Verification items for the finished model (mm, model axes). A direction names the side the tool comes from. Coordinates: 2 decimals unless noted, no trailing zeros. Order: outer loops, then holes, each group sorted by start corner. A loop starts at its lowest first (then second) coordinate and runs counter-clockwise, first axis right, second up. Notation, with made-up numbers: M 48,51 L 54,51 A10 ccw 54,66 Z; hole C 66,-8 d8. An arc over 180 degrees is marked long. Return JSON: item names as keys, results as strings. Group by question number.
1. Set-up check for faces 1 (the cylindrical face through (-0.867, -3.905, 69.451)), 2 (the cylindrical face through (-6.466, -2.681, 1.972)): record each of +Z, -Z, +X, -X, +Y, -Y from which the full face is reachable in a straight line by a thin tool's end or side.
2. Section check D-D, the plane z = 61. Record the cut outline in (x, y), plus the area to 3 significant figures.
3. Section check C-C, the plane z = 48. Record the cut outline in (x, y).
4. Gauge pin test, flat ends, axial feed: pin 1 (6 mm diameter, centred on x = 4, y = -0.5, fed in from +Z); pin 2 (2 mm diameter, centred on x = 2, z = 65.5, fed in from -Y); pin 3 (1 mm diameter, centred on x = -4, z = 39, fed in from +Y); pin 4 (5 mm diameter, centred on y = -0.5, z = 58, fed in from +X). Record the tip position at first contact, or that the pin passes through.
5. Section check A-A, the plane y = 0. Record the cut outline in (x, z).
6. Material ranges on line 1 along Z through (x, y) = (1.5, -5); line 2 along Y through (x, z) = (-0.25, 9.5); line 3 along Z through (x, y) = (3.5, -6), recorded low to high.
```python
from build123d import *

# Parameters (mm, degrees)
SKETCH1_R      = 5.5
EXTRUDE1_DEPTH = 66
EXTRUDE2_START = -9
SKETCH3_R      = 5.5
SKETCH3_R_2    = 4.5
EXTRUDE2_DEPTH = 9
SKETCH4_R      = 7
EXTRUDE3_DEPTH = 4
SKETCH5_R      = 4
EXTRUDE4_DEPTH = 7


with BuildPart() as part:
    # Sketch1 → Extrude1 (new body)
    with BuildSketch(Plane.XY):
        Circle(SKETCH1_R)
    extrude(amount=EXTRUDE1_DEPTH)

    # Sketch3 → Extrude2 (cut)
    with BuildSketch(Plane.XY.offset(66).offset(EXTRUDE2_START)):
        Circle(SKETCH3_R)
        Circle(SKETCH3_R_2, mode=Mode.SUBTRACT)
    extrude(amount=EXTRUDE2_DEPTH, mode=Mode.SUBTRACT)

    # Sketch4 → Extrude3 (add)
    with BuildSketch(Plane(origin=(0, 0, 0), x_dir=(-1, 0, 0), z_dir=(0, 0, -1))):
        Circle(SKETCH4_R)
    extrude(amount=-EXTRUDE3_DEPTH)

    # Sketch5 → Extrude4 (add)
    with BuildSketch(Plane.XY.offset(66)):
        Circle(SKETCH5_R)
    extrude(amount=EXTRUDE4_DEPTH)


solid = part.part
```
Answers follow:
{
 "1": {"face 1": "+Z", "face 2": "+Z, -Z"},
 "2": {"outline": "C 0,0 d9", "area": "63.6 mm^2"},
 "3": {"outline": "C 0,0 d11"},
 "4": {"pin 1": "z = 73", "pin 2": "y = -4.39", "pin 3": "y = 4.24", "pin 4": "x = 5.5"},
 "5": {"outline": "M -7,0 L 7,0 L 7,4 L 5.5,4 L 5.5,57 L 4.5,57 L 4.5,66 L 4,66 L 4,73 L -4,73 L -4,66 L -4.5,66 L -4.5,57 L -5.5,57 L -5.5,4 L -7,4 Z"},
 "6": {"line 1": "0 to 57", "line 2": "-5.49 to 5.49", "line 3": "0 to 4"}
}
